```python
from build123d import *

# Parameters (mm, degrees)
SKETCH_1_W          = 55
SKETCH_1_H          = 30
EXTRUDE_1_DEPTH     = 30
SKETCH_2_R          = 1.65
SKETCH_2_W          = 17
SKETCH_2_H          = 24
CUT_EXTRUDE_1_DEPTH = 40
CUT_EXTRUDE_3_DEPTH = 40
CUT_EXTRUDE_4_DEPTH = 6
CUT_EXTRUDE_5_DEPTH = 6
FILLET_1_R          = 2
FILLET_2_R          = 2
FILLET_3_R          = 2
SKETCH_10_R         = 1.65
CUT_EXTRUDE_7_DEPTH = 8
CUT_EXTRUDE_START   = -8
SKETCH_11_R         = 1.65
CUT_EXTRUDE_8_DEPTH = 8


with BuildPart() as part:
    # 草图1 → 凸台-拉伸1 (new body)
    with BuildSketch(Plane.XY):
        Rectangle(SKETCH_1_W, SKETCH_1_H)
    extrude(amount=EXTRUDE_1_DEPTH)

    # 草图2 → 切除-拉伸1 (cut)
    with BuildSketch(Plane(origin=(0, 15, 0), x_dir=(1, 0, 0), z_dir=(0, 1, 0))):
        with Locations(Location((12.5, -25, 0), (0, 0, 270))):
            Circle(SKETCH_2_R)
        with Locations(Location((-12.5, -25, 0), (0, 0, 270))):
            Circle(SKETCH_2_R)
        with Locations(Location((-12.5, -15, 0), (0, 0, 270))):
            Circle(SKETCH_2_R)
        with Locations(Location((12.5, -15, 0), (0, 0, 270))):
            Circle(SKETCH_2_R)
        with Locations((0, -15)):
            Rectangle(SKETCH_2_W, SKETCH_2_H)
    extrude(amount=-CUT_EXTRUDE_1_DEPTH, mode=Mode.SUBTRACT)

    # 草图7 → 切除-拉伸3 (cut)
    with BuildSketch(Plane(origin=(0, 15, 0), x_dir=(1, 0, 0), z_dir=(0, 1, 0))):
        Polygon((27.5, -15), (27.5, -30), (14.5, -30), align=None)
        Polygon((-14.5, -30), (-27.5, -30), (-27.5, -15), align=None)
    extrude(amount=-CUT_EXTRUDE_3_DEPTH, mode=Mode.SUBTRACT)

    # 草图8 → 切除-拉伸4 (cut)
    with BuildSketch(Plane(origin=(0, 15, 0), x_dir=(1, 0, 0), z_dir=(0, 1, 0))):
        Polygon((-16, -25.215471809), (-16, -11.5), (-10.5, -11.5), (-10.5, -2), (-25.5, -2), (-25.5, -14.253933347), align=None)
        Polygon((16, -25.215471809), (16, -11.5), (10.5, -11.5), (10.5, -2), (25.5, -2), (25.5, -14.253933347), align=None)
    extrude(amount=-CUT_EXTRUDE_4_DEPTH, mode=Mode.SUBTRACT)

    # 草图9 → 切除-拉伸5 (cut)
    with BuildSketch(Plane.XZ.offset(15)):
        Polygon((-16, 25.215471809), (-16, 11.5), (-10.5, 11.5), (-10.5, 2), (-25.5, 2), (-25.5, 14.253933347), align=None)
        Polygon((16.668372364, 24.444272927), (16, 11.5), (10.5, 11.5), (10.5, 2), (25.5, 2), (25.5, 14.253933347), align=None)
    extrude(amount=-CUT_EXTRUDE_5_DEPTH, mode=Mode.SUBTRACT)

    # 圆角1
    fillet_1_edges = [part.edges().sort_by_distance(p)[0] for p in [
        (-25.5, -12, 14.253933347),
        (-16, -12, 25.215471809),
        (-16, -12, 11.5),
        (-10.5, -12, 11.5),
        (-10.5, -12, 2),
        (-25.5, -12, 2),
        (25.5, -12, 2),
        (10.5, -12, 2),
        (10.5, -12, 11.5),
        (16, -12, 11.5),
        (16.668372364, -12, 24.444272927),
        (25.5, -12, 14.253933347),
        (8.5, 0, 3),
        (8.5, 0, 27),
        (-8.5, 0, 27),
        (-8.5, 0, 3),
    ]]
    fillet(fillet_1_edges, radius=FILLET_1_R)

    # 圆角2
    fillet_2_edges = [part.edges().sort_by_distance(p)[0] for p in [
        (25.5, 12, 14.253933347),
        (16, 12, 25.215471809),
        (16, 12, 11.5),
        (10.5, 12, 11.5),
        (10.5, 12, 2),
        (25.5, 12, 2),
        (-16, 12, 25.215471809),
        (-25.5, 12, 14.253933347),
        (-25.5, 12, 2),
        (-10.5, 12, 2),
        (-10.5, 12, 11.5),
        (-16, 12, 11.5),
    ]]
    fillet(fillet_2_edges, radius=FILLET_2_R)

    # 圆角3
    fillet_3_edges = [part.edges().sort_by_distance(p)[0] for p in [
        (-27.5, 0, 0),
        (-14.5, 0, 30),
        (14.5, 0, 30),
        (27.5, 0, 0),
        (27.5, 0, 15),
        (-27.5, 0, 15),
    ]]
    fillet(fillet_3_edges, radius=FILLET_3_R)

    # 草图10 → 切除-拉伸7 (cut)
    with BuildSketch(Plane.ZY.offset(27.5)):
        with Locations(Location((12, -6, 0), (0, 0, 270))):
            Circle(SKETCH_10_R)
        with Locations(Location((4, -6, 0), (0, 0, 270))):
            Circle(SKETCH_10_R)
        with Locations(Location((4, 6, 0), (0, 0, 270))):
            Circle(SKETCH_10_R)
        with Locations(Location((12, 6, 0), (0, 0, 270))):
            Circle(SKETCH_10_R)
    extrude(amount=-CUT_EXTRUDE_7_DEPTH, mode=Mode.SUBTRACT)

    # 草图11 → 切除-拉伸8 (cut)
    with BuildSketch(Plane(origin=(27.5, 0, 0), x_dir=(0, 0, -1), z_dir=(1, 0, 0)).offset(CUT_EXTRUDE_START)):
        with Locations(Location((-12, 6, 0), (0, 0, 270))):
            Circle(SKETCH_11_R)
        with Locations(Location((-4, 6, 0), (0, 0, 270))):
            Circle(SKETCH_11_R)
        with Locations(Location((-4, -6, 0), (0, 0, 270))):
            Circle(SKETCH_11_R)
        with Locations(Location((-12, -6, 0), (0, 0, 270))):
            Circle(SKETCH_11_R)
    extrude(amount=CUT_EXTRUDE_8_DEPTH, mode=Mode.SUBTRACT)


solid = part.part
```
Read the model definition and answer for the solid it produces. Units are mm, in the model's axes. A direction names the side the tool comes from. Coordinates: 2 decimals unless noted, no trailing zeros. Write each loop counter-clockwise with the first axis right and the second up, starting at its lowest first coordinate (ties: lowest second). Pieces come first, ordered by that corner, then holes. Notation, with made-up numbers: (67.5, -16.5) - (81.5, -16.5) arc R21 cw to (81.5, -8.5) - close; hole circle Ø5 at (38.5, -1). An arc over 180 degrees is marked (long way). Answer as a JSON object with one key per item and string values. Group by question number.
1. A cutting plane is placed at A-A (x = 3.5). Determine the outline of the cut face in (y, z), plus the area to 3 significant figures.
2. The mould has two halves that part along Z. Classify faces 6 (the cylindrical face through (-11.07, -11.96, 2.6)), 7 (the cylindrical face through (-26.9, 0.21, 0.57)), 8 (the flat face through (21, 0.2, 22.5)): +Z half, -Z half, draft (parallel to the pull), parting line (faces both ways), or undercut.
3. A cutting plane is placed at D-D (x = 11.5). Determine the outline of the cut face in (y, z), plus the area to 3 significant figures.
4. Which of the six approach directions +Z, -Z, +X, -X, +Y, -Y give full straight-line access (tool end or side, diameter ignored) to faces 1 (the cylindrical face through (23.44, 7.31, 5)), 2 (the cylindrical face through (-23.56, 7.65, 4.07)), 3 (the flat face through (18, 9, 10)), 4 (the cylindrical face through (26.9, 0.21, 0.57)), 5 (the cylindrical face through (-25.377, -11.958, 14.198))?
5. Consider L1, parallel to Y at x = 25.25, z = 12; L2, parallel to Z at x = 5, y = -6; L3, parallel to X at y = 2, z = 10.25. Determine where each line is inside the solid, lowest interval first. Write a range as [from, to].
6. A cutting plane is placed at C-C (z = 18). Determine the outline of the cut face in (x, y), plus the area to 3 significant figures.
7. Each of these flat-tipped pins is pushed along its axis until it touches: P1, Ø3, axis at x = -20, y = 11, coming from the +Z side; P2, Ø3, axis at y = -13, z = 17, coming from the -X side; P3, Ø1, axis at y = 5.5, z = 12.5, coming from the -X side; P4, Ø2, axis at x = -12.5, z = 15, coming from the -Y side. Where does it stop, or does it pass through?
8. A cutting plane is placed at B-B (y = 3.25). Determine the outline of the cut face in (x, z), plus the area to 3 significant figures.
Worked out:
{
 "1": {"outline": "(-15, 0) - (15, 0) - (15, 3) - (-15, 3) - close; (-15, 27) - (15, 27) - (15, 30) - (-15, 30) - close", "area": "180 mm²"},
 "2": {"face 6": "undercut", "face 7": "-Z half", "face 8": "+Z half"},
 "3": {"outline": "(-15, 0) - (15, 0) - (15, 2.27) - (9, 2.27) - (9, 11.23) - (15, 11.23) - (15, 13.69) - (-15, 13.69) - (-15, 11.23) - (-9, 11.23) - (-9, 2.27) - (-15, 2.27) - close; (-15, 16.31) - (15, 16.31) - (15, 23.69) - (-15, 23.69) - close; (-15, 26.31) - (15, 26.31) - (15, 30) - (-15, 30) - close", "area": "635 mm²"},
 "4": {"face 1": "+X", "face 2": "-X", "face 3": "+Y", "face 4": "-Z, +X, +Y, -Y", "face 5": "-Y"},
 "5": {"L1": "y = [-9, -7.65], [-4.35, 4.35], [7.65, 9]", "L2": "z = [0, 3], [27, 30]", "L3": "x = [-27.5, -8.5], [8.5, 27.5]"},
 "6": {"outline": "(-24.9, -15) - (-22.25, -15) - (-22.25, -9) - (-16, -9) - (-16, -15) - (-8.5, -15) - (-8.5, 15) - (-16, 15) - (-16, 9) - (-22.25, 9) - (-22.25, 15) - (-24.9, 15) - close; (8.5, -15) - (16.34, -15) - (16.34, -9) - (22.25, -9) - (22.25, -15) - (24.9, -15) - (24.9, 15) - (22.25, 15) - (22.25, 9) - (16, 9) - (16, 15) - (8.5, 15) - close", "area": "836 mm²"},
 "7": {"P1": "stops at z = 25.38", "P2": "stops at x = -27.06", "P3": "stops at x = -19.5", "P4": "passes through"},
 "8": {"outline": "(-27.5, 2) arc R2 ccw to (-25.5, 0) - (25.5, 0) arc R2 ccw to (27.5, 2) - (27.5, 14.25) arc R2 ccw to (27.01, 15.56) - (15.1, 29.31) arc R2 ccw to (13.59, 30) - (-13.59, 30) arc R2 ccw to (-15.1, 29.31) - (-27.01, 15.56) arc R2 ccw to (-27.5, 14.25) - close; hole circle Ø3.3 at (-12.5, 15); hole circle Ø3.3 at (-12.5, 25); hole (-8.5, 5) arc R2 ccw to (-6.5, 3) - (6.5, 3) arc R2 ccw to (8.5, 5) - (8.5, 25) arc R2 ccw to (6.5, 27) - (-6.5, 27) arc R2 ccw to (-8.5, 25) - close; hole circle Ø3.3 at (12.5, 15); hole circle Ø3.3 at (12.5, 25)", "area": "1,010 mm²"}
}
